```python
from build123d import *

# Parameters (mm, degrees)
SKETCH1_R           = 187.5
BOSS_EXTRUDE1_DEPTH = 250
SKETCH2_R           = 125
BOSS_EXTRUDE2_DEPTH = 500
FILLET1_R           = 15
FILLET2_R           = 20
CUT_EXTRUDE1_DEPTH  = 150


with BuildPart() as part:
    # Sketch1 → Boss-Extrude1 (new body)
    with BuildSketch(Plane(origin=(0, 0, 0), x_dir=(1, 0, 0), z_dir=(0, 1, 0))):
        with Locations(Location((0, 0, 0), (0, 0, 270))):
            Circle(SKETCH1_R)
    extrude(amount=BOSS_EXTRUDE1_DEPTH)

    # Sketch2 → Boss-Extrude2 (add)
    with BuildSketch(Plane(origin=(0, 250, 0), x_dir=(1, 0, 0), z_dir=(0, 1, 0))):
        with Locations(Location((0, 0, 0), (0, 0, 270))):
            Circle(SKETCH2_R)
    extrude(amount=BOSS_EXTRUDE2_DEPTH)

    # Fillet1
    fillet1_edges = [part.edges().sort_by_distance(p)[0] for p in [
        (0, 250, -125),
    ]]
    fillet(fillet1_edges, radius=FILLET1_R)

    # Fillet2
    fillet2_edges = [part.edges().sort_by_distance(p)[0] for p in [
        (0, 750, -125),
    ]]
    fillet(fillet2_edges, radius=FILLET2_R)

    # Sketch3 → Cut-Extrude1 (cut)
    with BuildSketch(Plane(origin=(0, 0, 0), x_dir=(-1, 0, 0), z_dir=(0, -1, 0))):
        Polygon((97.214244703, -31.619988955), (75.990836054, 68.380011045), (-21.223408649, 100), (-97.214244703, 31.619988955), (-75.990836054, -68.380011045), (21.223408649, -100), align=None)
    extrude(amount=-CUT_EXTRUDE1_DEPTH, mode=Mode.SUBTRACT)


solid = part.part
```
Geometry: final body of the model. Coordinates: model frame, mm. A direction names the side the tool comes from. Round coordinates to 2 decimals unless told otherwise and drop trailing zeros. Order: outer loops, then holes, each group sorted by start corner. A loop starts at its lowest first (then second) coordinate and runs counter-clockwise, first axis right, second up. Notation, with made-up numbers: (52.5, 10) - (91.5, 10) arc R32 cw to (91.5, 44) - close; hole circle Ø8 at (4.5, 74.25). An arc over 180 degrees is marked (long way). Use CSV: the item, a comma, the result in double quotes. Start each with the question number.
Q1. First-contact query: pin 1 (6 mm diameter, centred on y = 669, z = 106.5, fed in from +X); pin 2 (10 mm diameter, centred on x = 28.5, z = 91.5, fed in from -Y); pin 3 (5 mm diameter, centred on x = 57, y = 385.5, fed in from +Z); pin 4 (3 mm diameter, centred on x = 124, z = -92.5, fed in from +Y). Flat tips, straight axial feed; report the tip coordinate or a pass-through.
Q2. Section query D-D (y = 161.5). Return loops of the section in (x, z), and give its area (3 significant figures).
Q3. Section query C-C (y = 502). Return loops of the section in (x, z).
Q4. Mould query, pull axis X, two halves, no side actions, for faces 1 (the face through (5.5, 494.24, -124.88)), 2 (the face through (1, 150, -1)), 3 (the face through (1, 750, -1)). Classes: +X half, -X half, draft (parallel to the pull), parting line (faces both ways), or undercut.
Q5. Section query A-A (x = 0). Return loops of the section in (y, z), and give its area (3 significant figures).
Q6. Access query for faces 4 (the face through (44, 0, 81)), 5 (the face through (-13, 250, -140)), 6 (the face through (-58.687, 73.95, 66.289)). Directions: +Z, -Z, +X, -X, +Y, -Y. A direction counts if a zero-diameter tool reaches every point of the face in a straight line with its end or side. Return the directions, or none.
Q7. Section query B-B (z = 0). Return loops of the section in (x, y).
Q8. Material intervals for line 1 along Y through (x, z) = (127.5, 105.5); line 2 along Y through (x, z) = (-26.5, -42); line 3 along X through (y, z) = (185.5, 8), sorted ascending. Write a range as from..to.
Result set:
1,pin 1,"stops at x = 70.09"
1,pin 2,"stops at y = 0"
1,pin 3,"stops at z = 112.49"
1,pin 4,"stops at y = 250"
2,outline,"circle Ø375 at (0, 0)"
2,area,"110,000 mm2"
3,outline,"circle Ø250 at (0, 0)"
4,face 1,"parting line"
4,face 2,"undercut"
4,face 3,"draft"
5,outline,"(0, -187.5) - (250, -187.5) - (250, -140) arc R15 cw to (265, -125) - (730, -125) arc R20 ccw to (750, -105) - (750, 105) arc R20 ccw to (730, 125) - (265, 125) arc R15 cw to (250, 140) - (250, 187.5) - (0, 187.5) - (0, 93.1) - (150, 93.1) - (150, -93.1) - (0, -93.1) - close"
5,area,"191,000 mm2"
6,face 4,"+Z, -Z, +X, -X, -Y"
6,face 5,"+Y"
6,face 6,"-Y"
7,outline,"(-187.5, 0) - (-90.5, 0) - (-90.5, 150) - (90.5, 150) - (90.5, 0) - (187.5, 0) - (187.5, 250) - (140, 250) arc R15 cw to (125, 265) - (125, 730) arc R20 ccw to (105, 750) - (-105, 750) arc R20 ccw to (-125, 730) - (-125, 265) arc R15 cw to (-140, 250) - (-187.5, 250) - close"
8,line 1,"y = 0..250"
8,line 2,"y = 150..750"
8,line 3,"x = -187.33..187.33"
